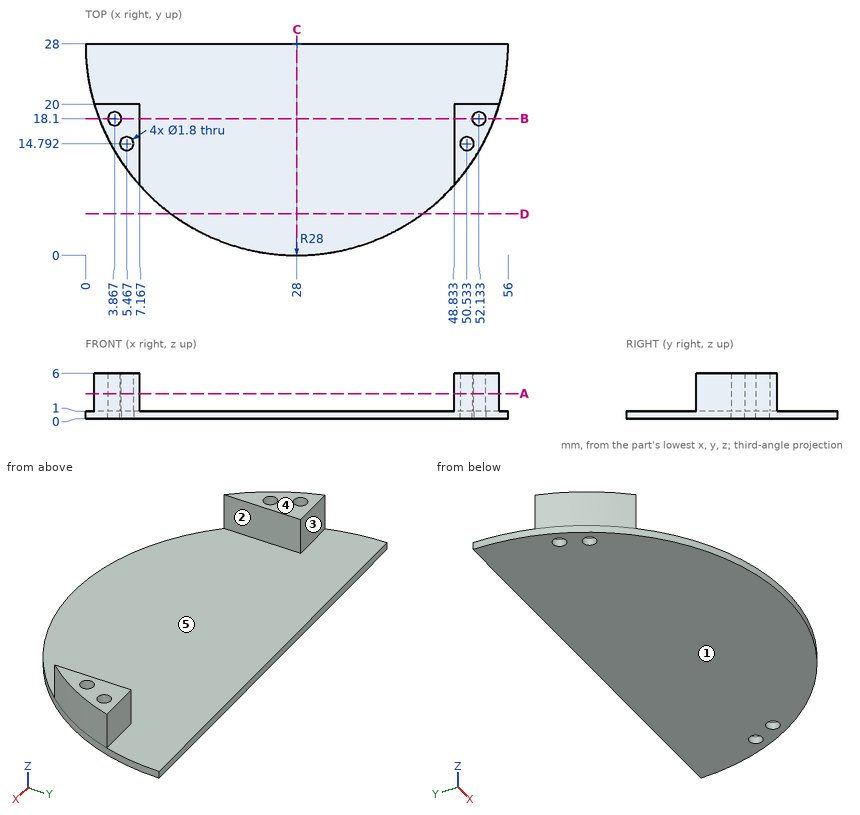
Can you work these out from the drawing? Everything is in mm from the part's minimum corner. A direction names the side the tool comes from. Coordinates: 2 decimals unless noted, no trailing zeros. Order: outer loops, then holes, each group sorted by start corner. A loop starts at its lowest first (then second) coordinate and runs counter-clockwise, first axis right, second up. Notation, with made-up numbers: M -19.5,49.25 L -15.5,49.25 A12 cw -15.5,66.25 Z; hole C 12.25,40 d7. An arc over 180 degrees is marked long. Answer as CSV lines item,"result". Start each with the question number.
1. I want a section at A-A, the plane z = 3.3. Write out the boundary of the cut face in (x, y).
2. I want a section at B-B, the plane y = 18.1. Write out the boundary of the cut face in (x, z).
3. On a 3-axis mill with a long thin cutter (end or side, diameter ignored), from which of +Z, -Z, +X, -X, +Y, -Y can I reach the whole of each face in a straight line? I mean the marked faces 1, 2 and 3. Say none if no direction works.
4. I want a section at D-D, the plane y = 5.5. Write out the boundary of the cut face in (x, z).
5. We'd pull the mould along X, two halves only. Please class the marked faces 4 and 5: released by +X, released by -X, zero draft, split by the parting line, or undercut.
6. I need wall thicknesses on line 1 (X direction, y = 14.25, z = 3.15) (1 decimal); line 2 (X direction, y = 18, z = 1.9); line 3 (X direction, y = 18.1, z = 0.5). Which ranges of each line are inside material? Lowest first, please. Write a range as [from, to].
7. I want a section at C-C, the plane x = 28. Write out the boundary of the cut face in (y, z), and give its area (3 significant figures).
8. For pin 1 (1 mm diameter, centred on y = 12, z = 0.5, fed in from +X); pin 2 (2 mm diameter, centred on y = 9.5, z = 2.5, fed in from +X); pin 3 (1.5 mm diameter, centred on x = 51, z = 4, fed in from +Y), each with a flat end and sliding along its axis, tell me the tip position at first contact or that it passes through.
Recorded:
1,outline,"M 1.17,20 A28 ccw 7.17,9.29 L 7.17,20 Z; M 48.83,9.29 A28 ccw 54.83,20 L 48.83,20 Z; hole C 3.87,18.1 d1.8; hole C 5.47,14.79 d1.8; hole C 50.53,14.79 d1.8; hole C 52.13,18.1 d1.8"
2,outline,"M 1.81,0 L 2.97,0 L 2.97,6 L 1.81,6 Z; M 4.77,0 L 51.23,0 L 51.23,6 L 48.83,6 L 48.83,1 L 7.17,1 L 7.17,6 L 4.77,6 Z; M 53.03,0 L 54.19,0 L 54.19,6 L 53.03,6 Z"
3,face 1,"-Z, +X, -X, +Y, -Y"
3,face 2,"+Z, +Y, -Y"
3,face 3,"+Z, +X, -X, +Y"
4,outline,"M 11.33,0 L 44.67,0 L 44.67,1 L 11.33,1 Z"
5,face 4,"zero draft"
5,face 5,"undercut"
6,line 1,"x = [3.6, 4.7], [6.2, 7.2], [48.8, 49.8], [51.3, 52.4]"
6,line 2,"x = [1.85, 2.97], [4.76, 7.17], [48.83, 51.24], [53.03, 54.15]"
6,line 3,"x = [1.81, 2.97], [4.77, 51.23], [53.03, 54.19]"
7,outline,"M 0,0 L 28,0 L 28,1 L 0,1 Z"
7,area,"28.0 mm2"
8,pin 1,"stops at x = 51.32"
8,pin 2,"stops at x = 49.86"
8,pin 3,"stops at y = 20"
